The listing builds one solid part. Answer for the finished solid, in the listing's coordinates (mm). A direction names the side the tool comes from. Coordinates: 2 decimals unless noted, no trailing zeros. Write each loop counter-clockwise with the first axis right and the second up, starting at its lowest first coordinate (ties: lowest second). Pieces come first, ordered by that corner, then holes. Notation, with made-up numbers: M -3,87 L 39,87 A25 ccw 39,102 Z; hole C -8.5,12.25 d3. An arc over 180 degrees is marked long. Answer as CSV lines item,"result".
```python
from build123d import *

# Parameters (mm, degrees)
SKETCH1_R           = 1.5
BOSS_EXTRUDE1_DEPTH = 3
FILLET1_R           = 0.5
CUT_EXTRUDE1_DEPTH  = 3


with BuildPart() as part:
    # Sketch1 → Boss-Extrude1 (new body)
    with BuildSketch(Plane(origin=(0, 0, 0), x_dir=(1, 0, 0), z_dir=(0, 1, 0))):
        Polygon((0, 0), (49, 0), (49, -19), (19, -49), (0, -49), (0, -19), align=None)
        with Locations(Location((9.5, -9.5, 0), (0, 0, 270))):
            Circle(SKETCH1_R, mode=Mode.SUBTRACT)
        with Locations(Location((39, -9.5, 0), (0, 0, 270))):
            Circle(SKETCH1_R, mode=Mode.SUBTRACT)
        with Locations(Location((9.5, -39, 0), (0, 0, 270))):
            Circle(SKETCH1_R, mode=Mode.SUBTRACT)
        with Locations(Location((9.5, -29, 0), (0, 0, 270))):
            Circle(SKETCH1_R, mode=Mode.SUBTRACT)
        with Locations(Location((29, -9.5, 0), (0, 0, 270))):
            Circle(SKETCH1_R, mode=Mode.SUBTRACT)
    extrude(amount=BOSS_EXTRUDE1_DEPTH)

    # Fillet1
    fillet1_edges = [part.edges().sort_by_distance(p)[0] for p in [
        (0, 1.5, 0),
        (49, 1.5, 0),
        (49, 1.5, 19),
        (19, 1.5, 49),
        (0, 1.5, 49),
    ]]
    fillet(fillet1_edges, radius=FILLET1_R)

    # Sketch2 → Cut-Extrude1 (cut)
    with BuildSketch(Plane(origin=(0, 3, 0), x_dir=(1, 0, 0), z_dir=(0, 1, 0))):
        with BuildLine():
            Line((23.658427125, -19.622893219), (40.098932188, -19.622893219))
            ThreePointArc((40.098932188, -19.622893219), (40.560871954, -19.931551503), (40.452485579, -20.476446609))
            Line((40.452485579, -20.476446609), (32.232233047, -28.696699141))
            ThreePointArc((32.232233047, -28.696699141), (31.878679656, -28.843145751), (31.525126266, -28.696699141))
            Line((31.525126266, -28.696699141), (23.304873734, -20.476446609))
            ThreePointArc((23.304873734, -20.476446609), (23.196487358, -19.931551503), (23.658427125, -19.622893219))
        make_face()
        with BuildLine():
            Line((20.476446609, -23.304873734), (28.696699141, -31.525126266))
            ThreePointArc((28.696699141, -31.525126266), (28.843145751, -31.878679656), (28.696699141, -32.232233047))
            Line((28.696699141, -32.232233047), (20.476446609, -40.452485579))
            ThreePointArc((20.476446609, -40.452485579), (19.931551503, -40.560871954), (19.622893219, -40.098932188))
            Line((19.622893219, -40.098932188), (19.622893219, -23.658427125))
            ThreePointArc((19.622893219, -23.658427125), (19.931551503, -23.196487358), (20.476446609, -23.304873734))
        make_face()
    extrude(amount=-CUT_EXTRUDE1_DEPTH, mode=Mode.SUBTRACT)


solid = part.part
```
Q1. Find section C-C (y = 2.45). Give the vertices of the cut face in (x, z), and give its area (3 significant figures).
Output:
outline,"M 0,0.5 A0.5 ccw 0.5,0 L 48.5,0 A0.5 ccw 49,0.5 L 49,18.79 A0.5 ccw 48.85,19.15 L 19.15,48.85 A0.5 ccw 18.79,49 L 0.5,49 A0.5 ccw 0,48.5 Z; hole C 9.5,9.5 d3; hole C 9.5,29 d3; hole C 9.5,39 d3; hole M 19.62,23.66 A0.5 ccw 20.48,23.3 L 28.7,31.53 A0.5 ccw 28.7,32.23 L 20.48,40.45 A0.5 ccw 19.62,40.1 Z; hole M 23.3,20.48 A0.5 ccw 23.66,19.62 L 40.1,19.62 A0.5 ccw 40.45,20.48 L 32.23,28.7 A0.5 ccw 31.53,28.7 Z; hole C 29,9.5 d3; hole C 39,9.5 d3"
area,"1,740 mm2"
Q2. For faces 1 (the flat face through (19, 0, 19)), 2 (the flat face through (24.644, 1.521, 36.285)), determine the directions among +Z, -Z, +X, -X, +Y, -Y from which every point of the face is accessible in a straight line to the end or side of a thin tool.
Output:
face 1,"+Z, -Z, +X, -X, -Y"
face 2,"+Y, -Y"
Q3. Straight lines are drawn through the part: line 1 (X direction, y = 1.6, z = 9.5); line 2 (X direction, y = 2.25, z = 29); line 3 (X direction, y = 2.7, z = 10). For each, find the intervals that lie inside material, in ascending order.
Output:
line 1,"0 to 8, 11 to 27.5, 30.5 to 37.5, 40.5 to 49"
line 2,"0 to 8, 11 to 19.62, 26.17 to 39"
line 3,"0 to 8.09, 10.91 to 27.59, 30.41 to 37.59, 40.41 to 49"
Q4. Flat-ended cylindrical pins translate along their axes: pin 1 Ø1 at (x, y) = (30, 2) entering from +Z; pin 2 Ø1.8 at (x, z) = (9.5, 29) entering from -Y. Find the tip coordinate at first contact, or state that the pin passes through.
Output:
pin 1,"z = 38.5"
pin 2,"through"
Q5. Find section A-A (x = 9.5). Give the vertices of the cut face in (y, z).
Output:
outline,"M 0,0 L 3,0 L 3,8 L 0,8 Z; M 0,11 L 3,11 L 3,27.5 L 0,27.5 Z; M 0,30.5 L 3,30.5 L 3,37.5 L 0,37.5 Z; M 0,40.5 L 3,40.5 L 3,49 L 0,49 Z"
Q6. The mould has two halves that part along Z. Classify faces 3 (the flat face through (36.4, 1.52, 24.53)), 4 (the flat face through (0, 1, 24)), 5 (the flat face through (34, 1, 34)): pulls with the +Z half, pulls with the -Z half, needs draft (parallel to the pull), parting line crosses it, or undercut.
Output:
face 3,"undercut"
face 4,"needs draft"
face 5,"pulls with the +Z half"
Q7. Find section B-B (z = 9.5). Give the vertices of the cut face in (x, y).
Output:
outline,"M 0,0 L 8,0 L 8,3 L 0,3 Z; M 11,0 L 27.5,0 L 27.5,3 L 11,3 Z; M 30.5,0 L 37.5,0 L 37.5,3 L 30.5,3 Z; M 40.5,0 L 49,0 L 49,3 L 40.5,3 Z"
Q8. Find section D-D (z = 35.5). Give the vertices of the cut face in (x, y).
Output:
outline,"M 0,0 L 19.62,0 L 19.62,3 L 0,3 Z; M 25.43,0 L 32.5,0 L 32.5,3 L 25.43,3 Z"
